For this review, take the finished solid that the model builds, in its own axes (mm). Round coordinates to 2 decimals unless told otherwise and drop trailing zeros. Loops run counter-clockwise (first coordinate to the right, second up) from the corner with the lowest first, then second, coordinate; pieces in that order, holes last.
```python
from build123d import *

# Parameters (mm, degrees)
SKETCH_W     = 80
SKETCH_H     = 400
PAD_DEPTH    = 10
SKETCH001_R  = 4
POCKET_DEPTH = 10


with BuildPart() as part:
    # Sketch → Pad (new body)
    with BuildSketch(Plane.YZ):
        Rectangle(SKETCH_W, SKETCH_H)
    extrude(amount=PAD_DEPTH)

    # Sketch001 → Pocket (cut)
    with BuildSketch(Plane.YZ.offset(10)):
        with Locations((0, 180)):
            Circle(SKETCH001_R)
        with Locations((0, 164)):
            Circle(SKETCH001_R)
    extrude(amount=-POCKET_DEPTH, mode=Mode.SUBTRACT)


solid = part.part
```
(1) Add section A-A (z = 164). Give the boundary of the cut face in (x, y).
(2) For L1, parallel to Z at x = 7.5, y = 0; L2, parallel to Z at x = 8.5, y = -1; L3, parallel to Y at x = 5, z = 166.5, list the stretches that pass through material, from the lowest coordinate up.
(3) The part is to be moulded in two halves that separate along Y. For faces 1 (the flat face through (5, -1, -200)), 2 (the cylindrical face through (5.07, -0.521, 167.966)), 3 (the flat face through (5, -40, -3)), say which applies: pulls with the +Y half, pulls with the -Y half, needs draft (parallel to the pull), parting line crosses it, or undercut.
(4) Add section B-B (y = 0). Give the boundary of the cut face in (x, z).
(5) Insertion check: pin 1 Ø10.5 at (y, z) = (0, 180) entering from -X. The pin has a flat end and moves straight along its axis. Give the tip position at first contact, or say it passes through.
Outcome:
1. outline: (0, -40) - (10, -40) - (10, -4) - (0, -4) - close; (0, 4) - (10, 4) - (10, 40) - (0, 40) - close
2. L1: z = -200 to 160, 168 to 176, 184 to 200
2. L2: z = -200 to 160.13, 167.87 to 176.13, 183.87 to 200
2. L3: y = -40 to -3.12, 3.12 to 40
3. face 1: needs draft
3. face 2: undercut
3. face 3: pulls with the -Y half
4. outline: (0, -200) - (10, -200) - (10, 160) - (0, 160) - close; (0, 168) - (10, 168) - (10, 176) - (0, 176) - close; (0, 184) - (10, 184) - (10, 200) - (0, 200) - close
5. pin 1: stops at x = 0
